The drawing under review shows one solid part. Ordinate dimensions are in mm from its lowest x, y, z. Round coordinates to 2 decimals unless told otherwise and drop trailing zeros. Loops run counter-clockwise (first coordinate to the right, second up) from the corner with the lowest first, then second, coordinate; pieces in that order, holes last. Notation, with made-up numbers: (23, 84) -> (27, 84) arc R12 ccw to (27, 90) -> close; hole circle Ø8 at (-34.5, 56). An arc over 180 degrees is marked (long way). Use a Markdown table: item, result. Add a question column.
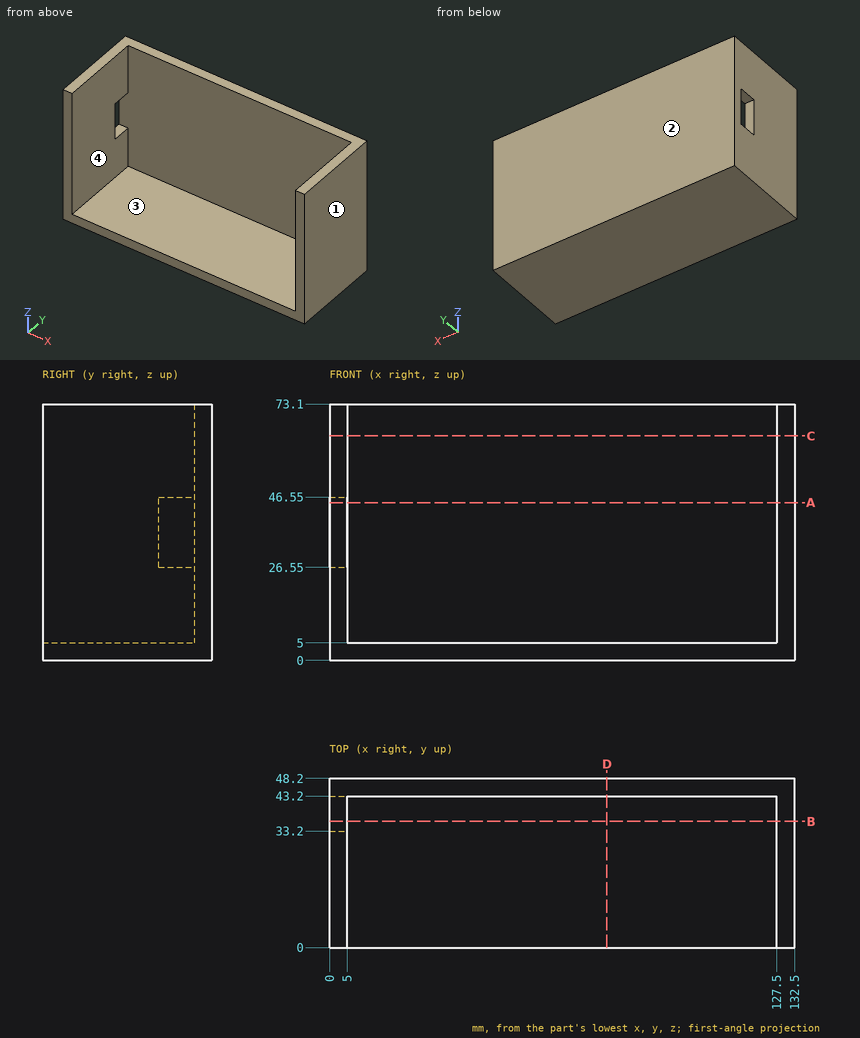
1. Mouldability with a two-part tool opening along X and no side actions: class the marked faces 1, 2, 3 and 4 as +X half, -X half, draft (parallel to the pull), parting line (faces both ways), or undercut.
2. Consider section D-D on x = 79. State the section outline as (y, z) points, plus the area to 4 significant figures.
3. Insertion check: P1, Ø1, axis at x = 59, y = 6, coming from the +Z side; P2, Ø4, axis at x = 87, z = 47.5, coming from the -Y side. Each pin has a flat end and moves straight along its axis. Give the tip position at first contact, or say it passes through.
4. Consider section C-C on z = 64. State the section outline as (x, y) points, plus the area to 3 significant figures.
5. To check wall thickness, follow probe 1 along X at (y, z) = (5, 16); probe 2 along Z at (x, y) = (51.5, 36); probe 3 along Y at (x, z) = (106, 20.5). State the ranges of each line that lie inside material, in increasing order. Write a range as from..to.
6. Consider section A-A on z = 45. State the section outline as (x, y) points, plus the area to 3 significant figures.
7. Consider section B-B on y = 36. State the section outline as (x, z) points.
Verdict:
| question | item | result |
|---|---|---|
| 1 | face 1 | +X half |
| 1 | face 2 | draft |
| 1 | face 3 | undercut |
| 1 | face 4 | undercut |
| 2 | outline | (0, 0) -> (48.2, 0) -> (48.2, 73.1) -> (43.2, 73.1) -> (43.2, 5) -> (0, 5) -> close |
| 2 | area | 581.5 mm² |
| 3 | P1 | stops at z = 5 |
| 3 | P2 | stops at y = 43.2 |
| 4 | outline | (0, 0) -> (5, 0) -> (5, 43.2) -> (127.5, 43.2) -> (127.5, 0) -> (132.5, 0) -> (132.5, 48.2) -> (0, 48.2) -> close |
| 4 | area | 1,090 mm² |
| 5 | probe 1 | x = 0..5, 127.5..132.5 |
| 5 | probe 2 | z = 0..5 |
| 5 | probe 3 | y = 43.2..48.2 |
| 6 | outline | (0, 0) -> (5, 0) -> (5, 33.2) -> (0, 33.2) -> close; (0, 43.2) -> (127.5, 43.2) -> (127.5, 0) -> (132.5, 0) -> (132.5, 48.2) -> (0, 48.2) -> close |
| 6 | area | 1,040 mm² |
| 7 | outline | (0, 0) -> (132.5, 0) -> (132.5, 73.1) -> (127.5, 73.1) -> (127.5, 5) -> (5, 5) -> (5, 26.55) -> (0, 26.55) -> close; (0, 46.55) -> (5, 46.55) -> (5, 73.1) -> (0, 73.1) -> close |
